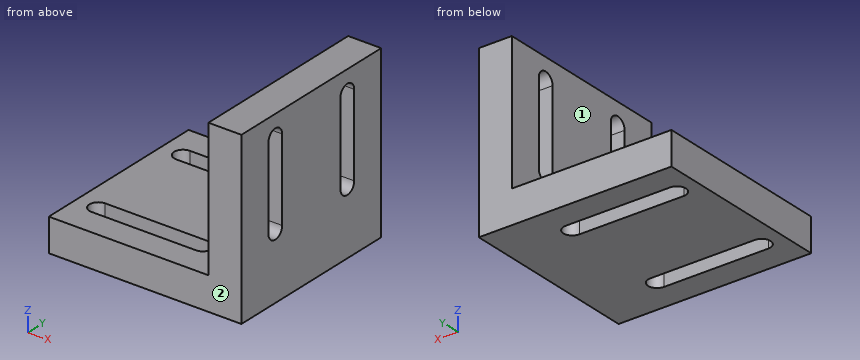
from build123d import *

# Parameters (mm, degrees)
SKETCH_1_W          = 70
SKETCH_1_H          = 66
EXTRUDE_1_DEPTH     = 12
SKETCH_2_W          = 12
SKETCH_2_H          = 66
EXTRUDE_2_DEPTH     = 50
CUT_EXTRUDE_1_DEPTH = 40
CUT_EXTRUDE_2_DEPTH = 40


with BuildPart() as part:
    # 草图1 → 凸台-拉伸1 (new body)
    with BuildSketch(Plane.XY):
        with Locations((35, 33)):
            Rectangle(SKETCH_1_W, SKETCH_1_H)
    extrude(amount=EXTRUDE_1_DEPTH)

    # 草图2 → 凸台-拉伸2 (add)
    with BuildSketch(Plane.XY.offset(12)):
        with Locations((64, 33)):
            Rectangle(SKETCH_2_W, SKETCH_2_H)
    extrude(amount=EXTRUDE_2_DEPTH)

    # 草图3 → 切除-拉伸1 (cut)
    with BuildSketch(Plane.ZY.offset(-58)):
        with BuildLine():
            Line((24, 19.25), (54, 19.25))
            ThreePointArc((54, 19.25), (57.25, 16), (54, 12.75))
            Line((54, 12.75), (24, 12.75))
            ThreePointArc((24, 12.75), (20.75, 16), (24, 19.25))
        make_face()
        with BuildLine():
            Line((24, 46.75), (54, 46.75))
            ThreePointArc((54, 46.75), (57.25, 50), (54, 53.25))
            Line((54, 53.25), (24, 53.25))
            ThreePointArc((24, 53.25), (20.75, 50), (24, 46.75))
        make_face()
    extrude(amount=-CUT_EXTRUDE_1_DEPTH, mode=Mode.SUBTRACT)

    # 草图6 → 切除-拉伸2 (cut)
    with BuildSketch(Plane.XY.offset(12)):
        with BuildLine():
            Line((8, 16.25), (46, 16.25))
            ThreePointArc((46, 16.25), (49.25, 13), (46, 9.75))
            Line((46, 9.75), (8, 9.75))
            ThreePointArc((8, 9.75), (4.75, 13), (8, 16.25))
        make_face()
        with BuildLine():
            Line((8, 49.75), (46, 49.75))
            ThreePointArc((46, 49.75), (49.25, 53), (46, 56.25))
            Line((46, 56.25), (8, 56.25))
            ThreePointArc((8, 56.25), (4.75, 53), (8, 49.75))
        make_face()
    extrude(amount=-CUT_EXTRUDE_2_DEPTH, mode=Mode.SUBTRACT)


solid = part.part
Source: CAD feature listing. Evaluate the final solid. Frame: model axes, mm. Face numbers are marked on the shaded views. A direction names the side the tool comes from. Coordinates: 2 decimals unless noted, no trailing zeros. Order: outer loops, then holes, each group sorted by start corner. A loop starts at its lowest first (then second) coordinate and runs counter-clockwise, first axis right, second up. Notation, with made-up numbers: M -22.75,-12.5 L 22.25,-12.5 A12 ccw 22.25,-0.5 Z; hole C 23.25,9 d11. An arc over 180 degrees is marked long. Write each question's results on one line, items separated by ' | '. Start each with the question number.
Item 1: Cut plane D-D (x = 52). Return loops of the section in (y, z).
Item 2: Line query: probe 1 along Y at (x, z) = (23.5, 3); probe 2 along Y at (x, z) = (63, 39); probe 3 along X at (y, z) = (20, 44.5). Output: solid intervals per line, ascending.
Item 3: Cut plane A-A (z = 48). Return loops of the section in (x, y).
Item 4: Cut plane C-C (y = 41.5). Return loops of the section in (x, z), and give its area (3 significant figures).
Item 5: Set-up query: the marked faces 1 and 2. Return all of +Z, -Z, +X, -X, +Y, -Y with unobstructed straight access to the full face (end or side cutting, diameter ignored); none if empty.
Item 6: Cut plane B-B (y = 11.5). Return loops of the section in (x, z).
Item 7: First-contact query: pin 1 Ø1.5 at (x, y) = (13.5, 17.5) entering from +Z; pin 2 Ø6 at (x, z) = (64.5, 37) entering from -Y; pin 3 Ø1 at (y, z) = (23, 18) entering from -X; pin 4 Ø6 at (x, z) = (29, 17) entering from +Y. Flat tips, straight axial feed; report the tip coordinate or a pass-through.
Checked values:
1) outline: M 0,0 L 66,0 L 66,12 L 0,12 Z
2) probe 1: y = 0 to 9.75, 16.25 to 49.75, 56.25 to 66 | probe 2: y = 0 to 12.75, 19.25 to 46.75, 53.25 to 66 | probe 3: x = 58 to 70
3) outline: M 58,0 L 70,0 L 70,12.75 L 58,12.75 Z; M 58,19.25 L 70,19.25 L 70,46.75 L 58,46.75 Z; M 58,53.25 L 70,53.25 L 70,66 L 58,66 Z
4) outline: M 0,0 L 70,0 L 70,62 L 58,62 L 58,12 L 0,12 Z | area: 1,440 mm2
5) face 1: +Z, -X, +Y, -Y | face 2: +Z, -Z, +X, -X, -Y
6) outline: M 0,0 L 5.12,0 L 5.12,12 L 0,12 Z; M 48.88,0 L 70,0 L 70,62 L 58,62 L 58,12 L 48.88,12 Z
7) pin 1: stops at z = 12 | pin 2: stops at y = 0 | pin 3: stops at x = 58 | pin 4: passes through
